The listing builds one solid part. Answer for the finished solid, in the listing's coordinates (mm). Face numbers are marked on the shaded views. A direction names the side the tool comes from. Round coordinates to 2 decimals unless told otherwise and drop trailing zeros. Write each loop counter-clockwise with the first axis right and the second up, starting at its lowest first coordinate (ties: lowest second). Pieces come first, ordered by that corner, then holes. Notation, with made-up numbers: (1, -25.5) -> (13, -25.5) arc R30 ccw to (13, 7.5) -> close; hole circle Ø5 at (-29.75, 4.5). An arc over 180 degrees is marked (long way). Write each question's results on one line, items separated by ' | '. Start each with the question number.
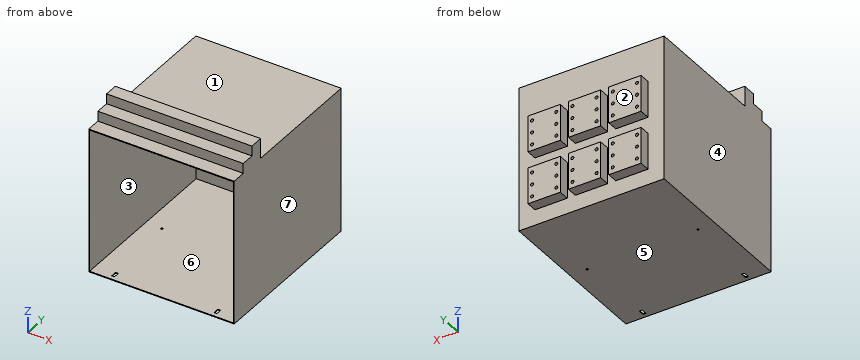
```python
from build123d import *

# Parameters (mm, degrees)
F0_W     = 523.494
F0_H     = 455.422
F1_DEPTH = 228.6
F2_T     = -2.54
F3_W     = 101.6
F3_H     = 114.3
F3_R     = 4.7625
F4_DEPTH = 34.036
F5_W     = 8.89
F5_H     = 19.05
F5_R     = 3.175
F6_DEPTH = 2.54
F8_DEPTH = 457.2


with BuildPart() as f1:
    # F0 (on Right) → F1 (new body, symmetric)
    with BuildSketch(Plane.YZ):
        Rectangle(F0_W, F0_H)
    extrude(amount=F1_DEPTH, both=True)

    # F2
    f2_openings = [f1.faces().sort_by_distance(p)[0] for p in [
        (0, -261.747, 0),
    ]]
    offset(amount=F2_T, openings=f2_openings)

    # F3 (on face) → F4 (join)
    with BuildSketch(Plane(origin=(0, 261.747, 0), x_dir=(-1, 0, 0), z_dir=(0, 1, 0))):
        with Locations((127, -121.539)):
            Rectangle(F3_W, F3_H)
        with Locations((88.9, -159.639)):
            Circle(F3_R, mode=Mode.SUBTRACT)
        with Locations((165.1, -159.639)):
            Circle(F3_R, mode=Mode.SUBTRACT)
        with Locations((88.9, -121.539)):
            Circle(F3_R, mode=Mode.SUBTRACT)
        with Locations((165.1, -121.539)):
            Circle(F3_R, mode=Mode.SUBTRACT)
        with Locations((88.9, -83.439)):
            Circle(F3_R, mode=Mode.SUBTRACT)
        with Locations((165.1, -83.439)):
            Circle(F3_R, mode=Mode.SUBTRACT)
        with Locations((127, 44.069)):
            Rectangle(F3_W, F3_H)
        with Locations((88.9, 5.969)):
            Circle(F3_R, mode=Mode.SUBTRACT)
        with Locations((165.1, 5.969)):
            Circle(F3_R, mode=Mode.SUBTRACT)
        with Locations((88.9, 44.069)):
            Circle(F3_R, mode=Mode.SUBTRACT)
        with Locations((165.1, 44.069)):
            Circle(F3_R, mode=Mode.SUBTRACT)
        with Locations((88.9, 82.169)):
            Circle(F3_R, mode=Mode.SUBTRACT)
        with Locations((165.1, 82.169)):
            Circle(F3_R, mode=Mode.SUBTRACT)
        with Locations((0, -121.539)):
            Rectangle(F3_W, F3_H)
        with Locations((-38.1, -159.639)):
            Circle(F3_R, mode=Mode.SUBTRACT)
        with Locations((-38.1, -121.539)):
            Circle(F3_R, mode=Mode.SUBTRACT)
        with Locations((-38.1, -83.439)):
            Circle(F3_R, mode=Mode.SUBTRACT)
        with Locations((38.1, -159.639)):
            Circle(F3_R, mode=Mode.SUBTRACT)
        with Locations((38.1, -121.539)):
            Circle(F3_R, mode=Mode.SUBTRACT)
        with Locations((38.1, -83.439)):
            Circle(F3_R, mode=Mode.SUBTRACT)
        with Locations((0, 44.069)):
            Rectangle(F3_W, F3_H)
        with Locations((-38.1, 5.969)):
            Circle(F3_R, mode=Mode.SUBTRACT)
        with Locations((-38.1, 44.069)):
            Circle(F3_R, mode=Mode.SUBTRACT)
        with Locations((-38.1, 82.169)):
            Circle(F3_R, mode=Mode.SUBTRACT)
        with Locations((38.1, 5.969)):
            Circle(F3_R, mode=Mode.SUBTRACT)
        with Locations((38.1, 44.069)):
            Circle(F3_R, mode=Mode.SUBTRACT)
        with Locations((38.1, 82.169)):
            Circle(F3_R, mode=Mode.SUBTRACT)
        with Locations((-127, -121.539)):
            Rectangle(F3_W, F3_H)
        with Locations((-165.1, -159.639)):
            Circle(F3_R, mode=Mode.SUBTRACT)
        with Locations((-165.1, -121.539)):
            Circle(F3_R, mode=Mode.SUBTRACT)
        with Locations((-88.9, -159.639)):
            Circle(F3_R, mode=Mode.SUBTRACT)
        with Locations((-88.9, -121.539)):
            Circle(F3_R, mode=Mode.SUBTRACT)
        with Locations((-165.1, -83.439)):
            Circle(F3_R, mode=Mode.SUBTRACT)
        with Locations((-88.9, -83.439)):
            Circle(F3_R, mode=Mode.SUBTRACT)
        with Locations((-127, 44.069)):
            Rectangle(F3_W, F3_H)
        with Locations((-165.1, 5.969)):
            Circle(F3_R, mode=Mode.SUBTRACT)
        with Locations((-88.9, 5.969)):
            Circle(F3_R, mode=Mode.SUBTRACT)
        with Locations((-165.1, 44.069)):
            Circle(F3_R, mode=Mode.SUBTRACT)
        with Locations((-165.1, 82.169)):
            Circle(F3_R, mode=Mode.SUBTRACT)
        with Locations((-88.9, 44.069)):
            Circle(F3_R, mode=Mode.SUBTRACT)
        with Locations((-88.9, 82.169)):
            Circle(F3_R, mode=Mode.SUBTRACT)
    extrude(amount=F4_DEPTH)

    # F5 (on face) → F6 (cut, through all)
    with BuildSketch(Plane(origin=(0, 0, -227.711), x_dir=(1, 0, 0), z_dir=(0, 0, -1))):
        with Locations((160.909, 238.76)):
            Rectangle(F5_W, F5_H)
        with Locations((-160.909, 238.76)):
            Rectangle(F5_W, F5_H)
        with Locations((174.244, -11.303)):
            Circle(F5_R)
        with Locations((-174.244, -11.303)):
            Circle(F5_R)
    extrude(amount=-F6_DEPTH, mode=Mode.SUBTRACT)

    # F7 (on face) → F8 (join, through all)
    with BuildSketch(Plane.YZ.offset(228.6)):
        Polygon((-217.297, 259.207), (-217.297, 227.711), (-132.461, 227.711), (-132.461, 290.703), (-174.879, 290.703), (-174.879, 259.207), align=None)
    extrude(amount=-F8_DEPTH)


solid = f1.part
```
Q1. For the marked faces 1, 2 and 3, determine the directions among +Z, -Z, +X, -X, +Y, -Y from which every point of the face is accessible in a straight line to the end or side of a thin tool.
Q2. Each of these flat-tipped pins is pushed along its axis until it touches: pin 1 (17 mm diameter, centred on x = 9.5, y = 270.5, fed in from +Z); pin 2 (12.5 mm diameter, centred on x = 38.1, z = 82.169, fed in from -Y); pin 3 (8.5 mm diameter, centred on x = -165.1, z = 82.169, fed in from +Y). Where does it stop, or does it pass through?
Q3. Find the intervals of material crossed by line 1 (X direction, y = 208.5, z = -113); line 2 (Z direction, x = -107, y = 238); line 3 (Z direction, x = 156.5, y = -185.5), in increasing order.
Q4. The part is cut by section D-D, the plane z = 169. Write down the section's boundary in (x, y).
Q5. The part is cut by section B-B, the plane z = 19. Write down the section's boundary in (x, y).
Q6. Determine the mould class of the marked faces 4, 5, 6 and 7 for opening direction X: pulls with the +X half, pulls with the -X half, needs draft (parallel to the pull), parting line crosses it, or undercut.
Q7. The part is cut by section A-A, the plane y = 249. Write down the section's boundary in (x, z), then the cut area to 3 significant figures.
Q8. The part is cut by section C-C, the plane x = 133.5. Write down the section's boundary in (y, z).
Answers follow:
1) face 1: +Z, +X, -X, +Y | face 2: +Z, -Z, +X, -X, +Y | face 3: -Y
2) pin 1: z = 101.22 | pin 2: y = 259.21 | pin 3: y = 261.75
3) line 1: -228.6 to -226.06, 226.06 to 228.6 | line 2: -227.71 to -225.17, 225.17 to 227.71 | line 3: -227.71 to -225.17, 225.17 to 259.21
4) outline: (-228.6, -261.75) -> (-226.06, -261.75) -> (-226.06, 259.21) -> (226.06, 259.21) -> (226.06, -261.75) -> (228.6, -261.75) -> (228.6, 261.75) -> (-228.6, 261.75) -> close
5) outline: (-228.6, -261.75) -> (-226.06, -261.75) -> (-226.06, 259.21) -> (226.06, 259.21) -> (226.06, -261.75) -> (228.6, -261.75) -> (228.6, 261.75) -> (177.8, 261.75) -> (177.8, 295.78) -> (76.2, 295.78) -> (76.2, 261.75) -> (50.8, 261.75) -> (50.8, 295.78) -> (-50.8, 295.78) -> (-50.8, 261.75) -> (-76.2, 261.75) -> (-76.2, 295.78) -> (-177.8, 295.78) -> (-177.8, 261.75) -> (-228.6, 261.75) -> close
6) face 4: pulls with the -X half | face 5: needs draft | face 6: undercut | face 7: pulls with the +X half
7) outline: (-228.6, -227.71) -> (228.6, -227.71) -> (228.6, 227.71) -> (-228.6, 227.71) -> close; hole (-226.06, -225.17) -> (226.06, -225.17) -> (226.06, 225.17) -> (-226.06, 225.17) -> close | area: 4,610 mm^2
8) outline: (-261.75, -227.71) -> (261.75, -227.71) -> (261.75, -178.69) -> (295.78, -178.69) -> (295.78, -64.39) -> (261.75, -64.39) -> (261.75, -13.08) -> (295.78, -13.08) -> (295.78, 101.22) -> (261.75, 101.22) -> (261.75, 227.71) -> (-132.46, 227.71) -> (-132.46, 290.7) -> (-174.88, 290.7) -> (-174.88, 259.21) -> (-217.3, 259.21) -> (-217.3, 227.71) -> (-261.75, 227.71) -> (-261.75, 225.17) -> (259.21, 225.17) -> (259.21, -225.17) -> (-261.75, -225.17) -> close
